Part model, mm, in its own coordinate system. A direction names the side the tool comes from. Coordinates: 2 decimals unless noted, no trailing zeros. Order: outer loops, then holes, each group sorted by start corner. A loop starts at its lowest first (then second) coordinate and runs counter-clockwise, first axis right, second up.
```python
from build123d import *

# Parameters (mm, degrees)
F0_W     = 1.25
F0_H     = 4
F0_W_2   = 1.75
F1_DEPTH = 6
F4_DEPTH = 4
F5_DEPTH = 4
F6_DEPTH = 4


# Not quite as in the source:
# - a feature names something its author has since deleted; it is built from what else it names


with BuildPart() as f1:
    # F0 (on Right) → F1 (new body)
    with BuildSketch(Plane.YZ):
        with Locations((-34.0711950026, -0.2365471814)):
            Rectangle(F0_W, F0_H)
        with Locations((-35.5711950026, -0.2365471814)):
            Rectangle(F0_W_2, F0_H)
        with BuildLine():
            Line((-38.1961950026, -2.2365471814), (-36.4461950026, -2.2365471814))
            Line((-36.4461950026, -2.2365471814), (-36.4461950026, 1.7634528186))
            Line((-36.4461950026, 1.7634528186), (-38.1961950026, 1.7634528186))
            Line((-38.1961950026, 1.7634528186), (-40.1961950026, 1.7634528186))
            ThreePointArc((-40.1961950026, 1.7634528186), (-41.9461950026, 0.0134528186), (-43.6961950026, 1.7634528186))
            Line((-43.6961950026, 1.7634528186), (-56.6961950026, 1.7634528186))
            Line((-56.6961950026, 1.7634528186), (-56.6961950026, -1.4865471814))
            Line((-56.6961950026, -1.4865471814), (-56.6961950026, -2.2365471814))
            Line((-56.6961950026, -2.2365471814), (-55.6961950026, -2.2365471814))
            Line((-55.6961950026, -2.2365471814), (-55.6961950026, -1.2365471814))
            Line((-55.6961950026, -1.2365471814), (-39.1961950026, -1.2365471814))
            Line((-39.1961950026, -1.2365471814), (-39.1961950026, -2.2365471814))
            Line((-39.1961950026, -2.2365471814), (-38.1961950026, -2.2365471814))
        make_face()
        with BuildLine():
            ThreePointArc((-43.6961950026, 1.7634528186), (-41.9461950026, 0.0134528186), (-40.1961950026, 1.7634528186))
            Line((-40.1961950026, 1.7634528186), (-41.1961950026, 1.7634528186))
            ThreePointArc((-41.1961950026, 1.7634528186), (-41.9461950026, 1.0134528186), (-42.6961950026, 1.7634528186))
            Line((-42.6961950026, 1.7634528186), (-43.6961950026, 1.7634528186))
        make_face()
        with BuildLine():
            Line((-41.1961950026, 1.7634528186), (-40.1961950026, 1.7634528186))
            ThreePointArc((-40.1961950026, 1.7634528186), (-41.9461950026, 3.5134528186), (-43.6961950026, 1.7634528186))
            Line((-43.6961950026, 1.7634528186), (-42.6961950026, 1.7634528186))
            ThreePointArc((-42.6961950026, 1.7634528186), (-41.9461950026, 2.5134528186), (-41.1961950026, 1.7634528186))
        make_face()
        Polygon((-56.6961950026, -1.4865471814), (-56.6961950026, 1.7634528186), (-58.4461950026, 1.7634528186), (-58.4461950026, -2.2365471814), (-56.6961950026, -2.2365471814), align=None)
        with Locations((-59.3211950026, -0.2365471814)):
            Rectangle(F0_W_2, F0_H)
        Polygon((-60.1961950026, -2.2365471814), (-60.1961950026, 1.7634528186), (-61.4461950026, 1.7634528186), (-61.4461950026, -0.2365471814), (-61.4461950026, -2.2365471814), align=None)
    extrude(amount=F1_DEPTH)

    # F2 (on face) → F4 (cut)
    with BuildSketch(Plane(origin=(0, 0, -2.2365471814), x_dir=(1, 0, 0), z_dir=(0, 0, -1))):
        with BuildLine():
            Line((0, 61.4461950026), (0, 58.9461950026))
            ThreePointArc((0, 58.9461950026), (0.732233047, 60.7139619556), (2.5, 61.4461950026))
            Line((2.5, 61.4461950026), (0, 61.4461950026))
        make_face()
        with BuildLine():
            ThreePointArc((3.5, 61.4461950026), (5.267766953, 60.7139619556), (6, 58.9461950026))
            Line((6, 58.9461950026), (6, 61.4461950026))
            Line((6, 61.4461950026), (3.5, 61.4461950026))
        make_face()
    extrude(amount=-F4_DEPTH, mode=Mode.SUBTRACT)

    # F2 (on face) → F5 (cut)
    with BuildSketch(Plane(origin=(0, 0, -2.2365471814), x_dir=(1, 0, 0), z_dir=(0, 0, -1))):
        with BuildLine():
            Line((1.25, 58.4407150745), (4.75, 58.4407150745))
            ThreePointArc((4.75, 58.4407150745), (3, 60.1907150745), (1.25, 58.4407150745))
        make_face()
        with BuildLine():
            ThreePointArc((1.25, 58.4407150745), (3, 56.6907150745), (4.75, 58.4407150745))
            Line((4.75, 58.4407150745), (1.25, 58.4407150745))
        make_face()
    extrude(amount=-F5_DEPTH, mode=Mode.SUBTRACT)

    # F3 (on face) → F6 (cut)
    with BuildSketch(Plane(origin=(0, 0, -2.2365471814), x_dir=(1, 0, 0), z_dir=(0, 0, -1))):
        with BuildLine():
            Line((1.25, 36.4720486104), (4.75, 36.4720486104))
            ThreePointArc((4.75, 36.4720486104), (3, 38.2220486104), (1.25, 36.4720486104))
        make_face()
        with BuildLine():
            Line((6, 33.4461950026), (6, 35.9461950026))
            ThreePointArc((6, 35.9461950026), (5.267766953, 34.1784280497), (3.5, 33.4461950026))
            Line((3.5, 33.4461950026), (6, 33.4461950026))
        make_face()
        with BuildLine():
            ThreePointArc((2.5, 33.4461950026), (0.732233047, 34.1784280497), (0, 35.9461950026))
            Line((0, 35.9461950026), (0, 33.4461950026))
            Line((0, 33.4461950026), (2.5, 33.4461950026))
        make_face()
        with BuildLine():
            ThreePointArc((1.25, 36.4720486104), (3, 34.7220486104), (4.75, 36.4720486104))
            Line((4.75, 36.4720486104), (1.25, 36.4720486104))
        make_face()
    extrude(amount=-F6_DEPTH, mode=Mode.SUBTRACT)


solid = f1.part
```
(1) Probe line 1 (Z direction, x = 5, y = -55.5); line 2 (X direction, y = -58.5, z = 0.1); line 3 (Y direction, x = 5.5, z = 2.1). List the from-to ranges inside material, lowest first.
(2) Slice it at B-B, the plane y = -35.5. Give the cut face in (x, z).
(3) Slice it at D-D, the plane x = 1. Give the cut face in (y, z), then the cut area to 3 significant figures.
(4) Slice it at C-C, the plane z = 0.65. Give the cut face in (x, y), then the cut area to 3 significant figures.
(5) Tool access for faces 1 (the face through (0.75, -34.16, -0.26)), 2 (the face through (3, -52, 1.763)), 3 (the face through (3, -48, -1.237)), 4 (the face through (2.3, -38.3, 1.763)): list every direction of +Z, -Z, +X, -X, +Y, -Y with a clear straight run to the whole face (end or side of a thin tool).
(6) Pull direction X, two halves, no side cores. Call faces 5 (the face through (5.25, -60.73, -0.26)), 6 (the face through (0, -48, 0)), 7 (the face through (3.38, -38.18, -0.26)), 8 (the face through (3.38, -60.15, -0.26)): +X half, -X half, draft (parallel to the pull), parting line (faces both ways), or undercut.
(7) Slice it at A-A, the plane x = 3.75. Give the cut face in (y, z).
(8) Drop flat-ended pins along their axis: pin 1 (0.8 mm diameter, centred on x = 4, z = -2, fed in from +Y); pin 2 (1.5 mm diameter, centred on x = 1, y = -48, fed in from +Z); pin 3 (3 mm diameter, centred on x = 3, y = -36.47, fed in from -Z); pin 4 (1.8 mm diameter, centred on x = 2, y = -44.5, fed in from -Z). Give the stop position or say it passes through.
Here are the results:
1. line 1: z = -1.24 to 1.76
1. line 2: x = 0 to 1.25, 4.75 to 6
1. line 3: y = -43.66 to -42.62, -41.28 to -40.23
2. outline: (0.04, -2.24) - (1.54, -2.24) - (1.54, 1.76) - (0.04, 1.76) - close; (4.46, -2.24) - (5.96, -2.24) - (5.96, 1.76) - (4.46, 1.76) - close
3. outline: (-60.95, -2.24) - (-55.7, -2.24) - (-55.7, -1.24) - (-39.2, -1.24) - (-39.2, -2.24) - (-33.95, -2.24) - (-33.95, 1.76) - (-40.2, 1.76) arc R1.75 ccw to (-43.7, 1.76) - (-60.95, 1.76) - close; hole circle Ø1.5 at (-41.95, 1.76)
3. area: 94.5 mm2
4. outline: (0, -58.95) arc R2.5 ccw to (2.5, -61.45) - (3.5, -61.45) arc R2.5 ccw to (6, -58.95) - (6, -35.95) arc R2.5 ccw to (3.5, -33.45) - (2.5, -33.45) arc R2.5 ccw to (0, -35.95) - close; hole circle Ø3.5 at (3, -58.44); hole circle Ø3.5 at (3, -36.47)
4. area: 143 mm2
5. face 1: +Z, -Z, -X, +Y
5. face 2: +Z, +X, -X, -Y
5. face 3: -Z, +X, -X
5. face 4: +Z, +X, -X, +Y
6. face 5: +X half
6. face 6: -X half
6. face 7: undercut
6. face 8: undercut
7. outline: (-61.43, -2.24) - (-60.02, -2.24) - (-60.02, 1.76) - (-61.43, 1.76) - close; (-56.86, -2.24) - (-55.7, -2.24) - (-55.7, -1.24) - (-39.2, -1.24) - (-39.2, -2.24) - (-38.05, -2.24) - (-38.05, 1.76) - (-40.2, 1.76) arc R1.75 ccw to (-43.7, 1.76) - (-56.86, 1.76) - close; (-34.89, -2.24) - (-33.46, -2.24) - (-33.46, 1.76) - (-34.89, 1.76) - close; hole circle Ø1.5 at (-41.95, 1.76)
8. pin 1: stops at y = -33.45
8. pin 2: stops at z = 1.76
8. pin 3: passes through
8. pin 4: stops at z = -1.24
